Autodesk Inventor part; units mm, degrees
ref_plane "YZ Plane" through (0, 0, 0) normal (1, 0, 0) x (0, 1, 0)
ref_plane "XZ Plane" through (0, 0, 0) normal (0, 1, 0) x (-1, 0, 0)
ref_plane "XY Plane" through (0, 0, 0) normal (0, 0, 1) x (1, 0, 0)
sketch "스케치1" plane through (0, 0, 0) normal (0, 0, 1) x (1, 0, 0)
  line L0 (0, 0) -> (20, 0)
  line L1 (20, 0) -> (20, -33.5)
  line L2 (20, -33.5) -> (0, -33.5)
  line L3 (0, -33.5) -> (0, 0)
  dimension "d0" = 33.5
  dimension "d1" = 20
extrude "돌출1" add sketch "스케치1" along normal blind 30
sketch "스케치2" plane through (0, 0, 0) normal (0, 0, -1) x (-1, 0, 0)
  circle A0 centre (-10, -18.5) radius 2
  line L0 (0, 0) -> (0, -33.5)
  line L1 (-20, 0) -> (0, 0)
  dimension "d4" = 4
  dimension "d5" = 10
  dimension "d6" = 18.5
extrude "돌출2" cut sketch "스케치2" against normal blind 100
properties part number "linear_actuator"
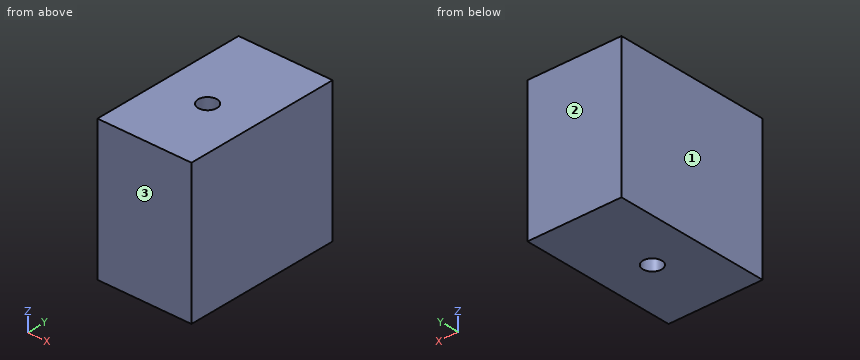
Work out the finished part from the listing and answer in its coordinate system (mm). Face numbers are marked on the shaded views. Round coordinates to 2 decimals unless told otherwise and drop trailing zeros. Write each loop counter-clockwise with the first axis right and the second up, starting at its lowest first coordinate (ties: lowest second). Pieces come first, ordered by that corner, then holes.
1) The mould has two halves that part along Y. Classify the marked faces 1, 2 and 3: pulls with the +Y half, pulls with the -Y half, needs draft (parallel to the pull), parting line crosses it, or undercut.
2) A cutting plane is placed at A-A (x = 10). Give the vertices of the cut face in (y, z), plus the area to 3 significant figures.
3) Straight lines are drawn through the part: line 1 (Y direction, x = 10, z = 14.75); line 2 (Y direction, x = 10.75, z = 11.5); line 3 (X direction, y = -19, z = 15.25). For each, find the intervals that lie inside material, in ascending order.
4) A cutting plane is placed at C-C (z = 2.5). Give the vertices of the cut face in (x, y), plus the area to 3 significant figures.
5) A cutting plane is placed at B-B (y = -18.5). Give the vertices of the cut face in (x, z).
Completed:
1. face 1: needs draft
1. face 2: pulls with the +Y half
1. face 3: pulls with the -Y half
2. outline: (-33.5, 0) - (-20.5, 0) - (-20.5, 30) - (-33.5, 30) - close; (-16.5, 0) - (0, 0) - (0, 30) - (-16.5, 30) - close
2. area: 885 mm2
3. line 1: y = -33.5 to -20.5, -16.5 to 0
3. line 2: y = -33.5 to -20.35, -16.65 to 0
3. line 3: x = 0 to 8.06, 11.94 to 20
4. outline: (0, -33.5) - (20, -33.5) - (20, 0) - (0, 0) - close; hole circle Ø4 at (10, -18.5)
4. area: 657 mm2
5. outline: (0, 0) - (8, 0) - (8, 30) - (0, 30) - close; (12, 0) - (20, 0) - (20, 30) - (12, 30) - close
